Could you check a few things on this model? Use its own coordinates, in mm. A direction names the side the tool comes from. Give positions to 0.01 mm unless a question says otherwise; leave off trailing zeros. Loops run counter-clockwise (first coordinate to the right, second up) from the corner with the lowest first, then second, coordinate; pieces in that order, holes last. Notation, with made-up numbers: (48.5, 20.25) - (87.5, 20.25) arc R7 ccw to (87.5, 27.25) - close; hole circle Ø9 at (16, 88). An arc over 180 degrees is marked (long way). Write each question's results on one line, items separated by ' | '. Start each with the question number.
1) I want a section at D-D, the plane x = 25. Write out the boundary of the cut face in (y, z).
2) I want a section at A-A, the plane z = -12.5. Write out the boundary of the cut face in (x, y), and give its area (3 significant figures).
3) I want a section at C-C, the plane y = 52.5. Write out the boundary of the cut face in (x, z), and give its area (3 significant figures).
4) If I drill on probe 1 along X at (y, z) = (52, 14); probe 2 along X at (y, z) = (20.5, -4); probe 3 along X at (y, z) = (17, -12.5), over which ranges is the centre line in solid material (lowest first)? Write a range as [from, to].
5) I'm going to push flat-ended pins straight in: pin 1 (1 mm diameter, centred on x = 21, z = 13, fed in from +Y); pin 2 (5 mm diameter, centred on x = -57.5, z = 12.5, fed in from -Y); pin 3 (5 mm diameter, centred on x = 45.5, z = 3.5, fed in from -Y); pin 4 (8 mm diameter, centred on x = -17, z = -11, fed in from +Y). Where does each tip first touch, or does it pass through?
6) On a 3-axis mill with a long thin cutter (end or side, diameter ignored), from which of +Z, -Z, +X, -X, +Y, -Y can I reach the whole of each face in a straight line? I mean faces 4 (the face through (-2, 58, 20)), 5 (the face through (19, 7, 7.5)), 6 (the face through (58.974, 2.465, 7.891)), 7 (the face through (56, 37.5, 0)). Say none if no direction works.
7) If we mould it in two halves opening along Z, with no side actions, what happens to faces 1 (the face through (55.1, 21.5, -8.7)), 2 (the face through (-1, 30, -22.5)), 3 (the face through (-1, 30, 22.5))? For each: +Z half, -Z half, draft (parallel to the pull), parting line (faces both ways), or undercut.
8) I want a section at B-B, the plane x = -57.5. Count the separate pieces of the cut face and the enclosed holes in it, and give its area (3 significant figures).
from build123d import *

# Parameters (mm, degrees)
SKETCH1_W           = 130
SKETCH1_H           = 45
BOSS_EXTRUDE1_DEPTH = 60
SHELL3_T            = -2.5
SKETCH4_W           = 2.5
SKETCH4_H           = 40
BOSS_EXTRUDE2_DEPTH = 57.5
SKETCH5_W           = 13
SKETCH5_H           = 40
BOSS_EXTRUDE3_DEPTH = 35
SKETCH6_W           = 20
SKETCH6_H           = 40
BOSS_EXTRUDE4_DEPTH = 20
SKETCH7_W           = 10
SKETCH7_H           = 40
BOSS_EXTRUDE5_DEPTH = 25
SKETCH9_R           = 1.5
CUT_EXTRUDE1_DEPTH  = 27.5
SKETCH11_R          = 1.5
CUT_EXTRUDE2_DEPTH  = 37.5
SKETCH16_W          = 20
SKETCH16_H          = 15
CUT_EXTRUDE3_DEPTH  = 2.5
SKETCH18_W          = 15
SKETCH18_H          = 10
CUT_EXTRUDE4_DEPTH  = 22.5
SKETCH19_W          = 40
SKETCH19_H          = 5
CUT_EXTRUDE5_DEPTH  = 2.5
SKETCH20_W          = 40
SKETCH20_H          = 5
CUT_EXTRUDE6_DEPTH  = 2.5
SKETCH21_R          = 3
CUT_EXTRUDE7_DEPTH  = 5
SKETCH22_W          = 127.5
SKETCH22_H          = 2
CUT_EXTRUDE8_DEPTH  = 1
SKETCH23_W          = 127.5
SKETCH23_H          = 2
CUT_EXTRUDE9_DEPTH  = 1


with BuildPart() as part:
    # Sketch1 → Boss-Extrude1 (new body)
    with BuildSketch(Plane(origin=(0, 0, 0), x_dir=(1, 0, 0), z_dir=(0, 1, 0))):
        Rectangle(SKETCH1_W, SKETCH1_H)
    extrude(amount=BOSS_EXTRUDE1_DEPTH)

    # Shell3
    shell3_openings = [part.faces().sort_by_distance(p)[0] for p in [
        (0, 60, 0),
    ]]
    offset(amount=SHELL3_T, openings=shell3_openings, kind=Kind.INTERSECTION)

    # Sketch4 → Boss-Extrude2 (add)
    with BuildSketch(Plane(origin=(0, 2.5, 0), x_dir=(1, 0, 0), z_dir=(0, 1, 0))):
        with Locations((28.75, 0)):
            Rectangle(SKETCH4_W, SKETCH4_H)
    extrude(amount=BOSS_EXTRUDE2_DEPTH)

    # Sketch5 → Boss-Extrude3 (add)
    with BuildSketch(Plane(origin=(0, 2.5, 0), x_dir=(1, 0, 0), z_dir=(0, 1, 0))):
        with Locations((56, 0)):
            Rectangle(SKETCH5_W, SKETCH5_H)
    extrude(amount=BOSS_EXTRUDE3_DEPTH)

    # Sketch6 → Boss-Extrude4 (add)
    with BuildSketch(Plane(origin=(0, 2.5, 0), x_dir=(1, 0, 0), z_dir=(0, 1, 0))):
        with Locations((17.5, 0)):
            Rectangle(SKETCH6_W, SKETCH6_H)
    extrude(amount=BOSS_EXTRUDE4_DEPTH)

    # Sketch7 → Boss-Extrude5 (add)
    with BuildSketch(Plane(origin=(0, 2.5, 0), x_dir=(1, 0, 0), z_dir=(0, 1, 0))):
        with Locations((-57.5, 0)):
            Rectangle(SKETCH7_W, SKETCH7_H)
    extrude(amount=BOSS_EXTRUDE5_DEPTH)

    # Sketch9 → Cut-Extrude1 (cut)
    with BuildSketch(Plane(origin=(0, 27.5, 0), x_dir=(1, 0, 0), z_dir=(0, 1, 0))):
        with Locations(Location((-57.5, 12.5, 0), (0, 0, 270))):
            Circle(SKETCH9_R)
        with Locations(Location((-57.5, -12.5, 0), (0, 0, 270))):
            Circle(SKETCH9_R)
    extrude(amount=-CUT_EXTRUDE1_DEPTH, mode=Mode.SUBTRACT)

    # Sketch11 → Cut-Extrude2 (cut)
    with BuildSketch(Plane(origin=(0, 37.5, 0), x_dir=(1, 0, 0), z_dir=(0, 1, 0))):
        with Locations(Location((56, 7.5, 0), (0, 0, 270))):
            Circle(SKETCH11_R)
        with Locations(Location((56, -7.5, 0), (0, 0, 270))):
            Circle(SKETCH11_R)
    extrude(amount=-CUT_EXTRUDE2_DEPTH, mode=Mode.SUBTRACT)

    # Sketch16 → Cut-Extrude3 (cut)
    with BuildSketch(Plane(origin=(-62.5, 0, 0), x_dir=(0, 0, -1), z_dir=(1, 0, 0))):
        with Locations((0, 35)):
            Rectangle(SKETCH16_W, SKETCH16_H)
    extrude(amount=-CUT_EXTRUDE3_DEPTH, mode=Mode.SUBTRACT)

    # Sketch18 → Cut-Extrude4 (cut)
    with BuildSketch(Plane.ZY.offset(-7.5)):
        with Locations((0, 7.5)):
            Rectangle(SKETCH18_W, SKETCH18_H)
    extrude(amount=-CUT_EXTRUDE4_DEPTH, mode=Mode.SUBTRACT)

    # Sketch19 → Cut-Extrude5 (cut)
    with BuildSketch(Plane(origin=(-62.5, 0, 0), x_dir=(0, 0, -1), z_dir=(1, 0, 0))):
        with Locations((0, 57.5)):
            Rectangle(SKETCH19_W, SKETCH19_H)
    extrude(amount=-CUT_EXTRUDE5_DEPTH, mode=Mode.SUBTRACT)

    # Sketch20 → Cut-Extrude6 (cut)
    with BuildSketch(Plane.ZY.offset(-27.5)):
        with Locations((0, 57.5)):
            Rectangle(SKETCH20_W, SKETCH20_H)
    extrude(amount=-CUT_EXTRUDE6_DEPTH, mode=Mode.SUBTRACT)

    # Sketch21 → Cut-Extrude7 (cut)
    with BuildSketch(Plane.XZ):
        with Locations(Location((56, -7.5, 0), (0, 0, 270))):
            Circle(SKETCH21_R)
        with Locations(Location((56, 7.5, 0), (0, 0, 270))):
            Circle(SKETCH21_R)
        with Locations(Location((-57.5, -12.5, 0), (0, 0, 270))):
            Circle(SKETCH21_R)
        with Locations(Location((-57.5, 12.5, 0), (0, 0, 270))):
            Circle(SKETCH21_R)
    extrude(amount=-CUT_EXTRUDE7_DEPTH, mode=Mode.SUBTRACT)

    # Sketch22 → Cut-Extrude8 (cut)
    with BuildSketch(Plane.XY.offset(-20)):
        with Locations((-1.25, 56)):
            Rectangle(SKETCH22_W, SKETCH22_H)
    extrude(amount=-CUT_EXTRUDE8_DEPTH, mode=Mode.SUBTRACT)

    # Sketch23 → Cut-Extrude9 (cut)
    with BuildSketch(Plane(origin=(0, 0, 20), x_dir=(-1, 0, 0), z_dir=(0, 0, -1))):
        with Locations((1.25, 56)):
            Rectangle(SKETCH23_W, SKETCH23_H)
    extrude(amount=-CUT_EXTRUDE9_DEPTH, mode=Mode.SUBTRACT)


solid = part.part
Answers:
1) outline: (0, -22.5) - (60, -22.5) - (60, -20) - (57, -20) - (57, -21) - (55, -21) - (55, -20) - (22.5, -20) - (22.5, 20) - (55, 20) - (55, 21) - (57, 21) - (57, 20) - (60, 20) - (60, 22.5) - (0, 22.5) - close; hole (2.5, -7.5) - (12.5, -7.5) - (12.5, 7.5) - (2.5, 7.5) - close
2) outline: (-65, 0) - (-60.5, 0) - (-60.5, 5) - (-59, 5) - (-59, 27.5) - (-62.5, 27.5) - (-62.5, 55) - (-65, 55) - close; (-56, 5) - (-54.5, 5) - (-54.5, 0) - (65, 0) - (65, 60) - (62.5, 60) - (62.5, 37.5) - (49.5, 37.5) - (49.5, 2.5) - (30, 2.5) - (30, 55) - (27.5, 55) - (27.5, 22.5) - (7.5, 22.5) - (7.5, 2.5) - (-52.5, 2.5) - (-52.5, 27.5) - (-56, 27.5) - close | area: 1,740 mm2
3) outline: (-65, -22.5) - (65, -22.5) - (65, 22.5) - (-65, 22.5) - close; hole (-62.5, -20) - (27.5, -20) - (27.5, 20) - (-62.5, 20) - close; hole (30, -20) - (62.5, -20) - (62.5, 20) - (30, 20) - close | area: 950 mm2
4) probe 1: x = [-65, -62.5], [27.5, 30], [62.5, 65] | probe 2: x = [-65, -52.5], [7.5, 30], [49.5, 65] | probe 3: x = [-65, -59], [-56, -52.5], [7.5, 30], [49.5, 65]
5) pin 1: stops at y = 22.5 | pin 2: stops at y = 5 | pin 3: stops at y = 0 | pin 4: stops at y = 2.5
6) face 4: -X, +Y | face 5: none | face 6: -Y | face 7: +Y
7) face 1: undercut | face 2: -Z half | face 3: +Z half
8) separate pieces: 3 | enclosed holes: 0 | area: 1,200 mm2
